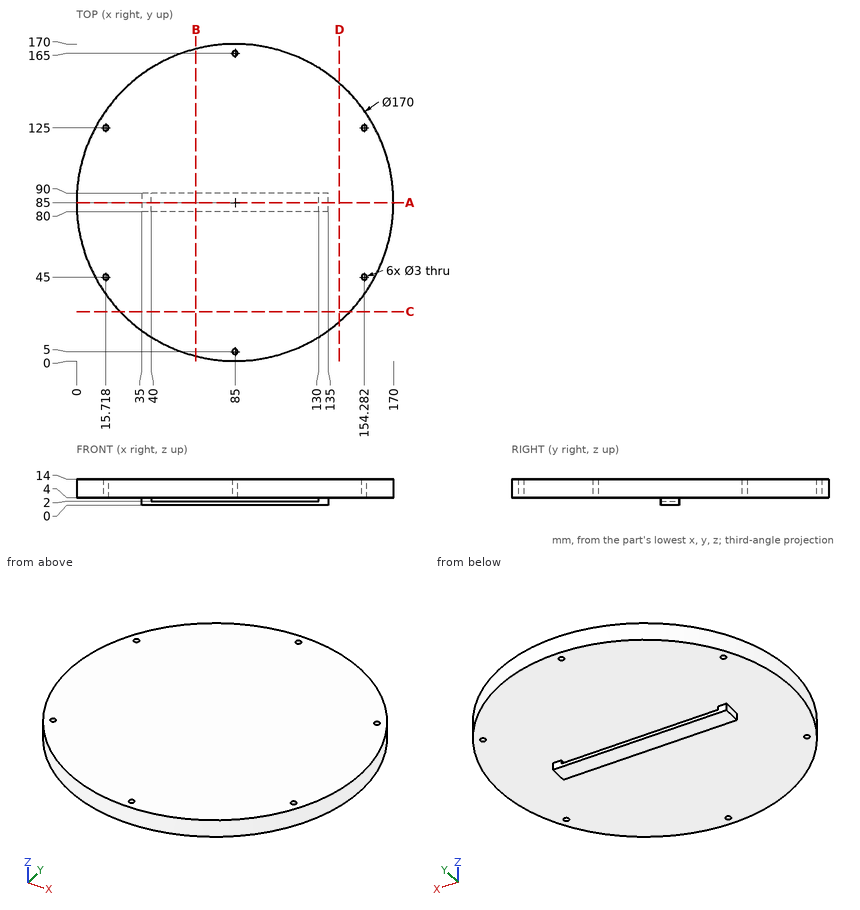
Design review of the part shown in the three views and the two pictorial views. Dimensions are in mm from the part's minimum x, y and z. Round coordinates to 2 decimals unless told otherwise and drop trailing zeros. Write each loop counter-clockwise with the first axis right and the second up, starting at its lowest first coordinate (ties: lowest second). Pieces come first, ordered by that corner, then holes. Notation, with made-up numbers: (63.5, 38) -> (80.5, 38) arc R13 ccw to (80.5, 42) -> close; hole circle Ø8 at (14.5, 21). An arc over 180 degrees is marked (long way). Write item = value, one per line. Start each with the question number.
1) Take a section at C-C, the plane y = 26.5. State the section outline as (x, z) points.
2) Take a section at B-B, the plane x = 64. State the section outline as (y, z) points (3 decimals).
3) Wall thickness on probe 1 along Y at (x, z) = (85, 6.5); probe 2 along X at (y, z) = (125, 9.5); probe 3 along Z at (x, y) = (15, 115.5): over which ranges is each line inside the solid? List them lowest first. Write a range as from..to.
4) Take a section at A-A, the plane y = 85. State the section outline as (x, z) points.
5) Clearance check with flat-ended pins moving along their axes: pin 1 (2.5 mm diameter, centred on x = 15.72, y = 45, fed in from +Z); pin 2 (1 mm diameter, centred on y = 85.5, z = 3, fed in from -X); pin 3 (3 mm diameter, centred on x = 30.5, y = 57.5, fed in from -Z); pin 4 (2 mm diameter, centred on y = 46, z = 11, fed in from +X). State where each tip first meets the part, or that it passes through.
6) Take a section at D-D, the plane x = 141. State the section outline as (y, z) points, plus the area to 3 significant figures.
Results list:
q1.outline = (23.33, 4) -> (146.67, 4) -> (146.67, 14) -> (23.33, 14) -> close
q2.outline = (2.635, 4) -> (167.365, 4) -> (167.365, 14) -> (2.635, 14) -> close; (80, 0) -> (90, 0) -> (90, 2) -> (80, 2) -> close
q3.probe_1 = 0..3.5, 6.5..163.5, 166.5..170
q3.probe_2 = 10..14.22, 17.22..152.78, 155.78..160
q3.probe_3 = 4..14
q4.outline = (0, 4) -> (35, 4) -> (35, 0) -> (135, 0) -> (135, 4) -> (170, 4) -> (170, 14) -> (0, 14) -> close; hole (40, 2) -> (130, 2) -> (130, 4) -> (40, 4) -> close
q5.pin_1 = through
q5.pin_2 = 35
q5.pin_3 = 4
q5.pin_4 = 161.03
q6.outline = (21.05, 4) -> (148.95, 4) -> (148.95, 14) -> (21.05, 14) -> close
q6.area = 1,280 mm²
